Input: part model. Units: mm. Frame: model coordinates. Give positions to 0.01 mm unless a question says otherwise; leave off trailing zeros. Write each loop counter-clockwise with the first axis right and the second up, starting at its lowest first coordinate (ties: lowest second). Pieces come first, ordered by that corner, then holes.
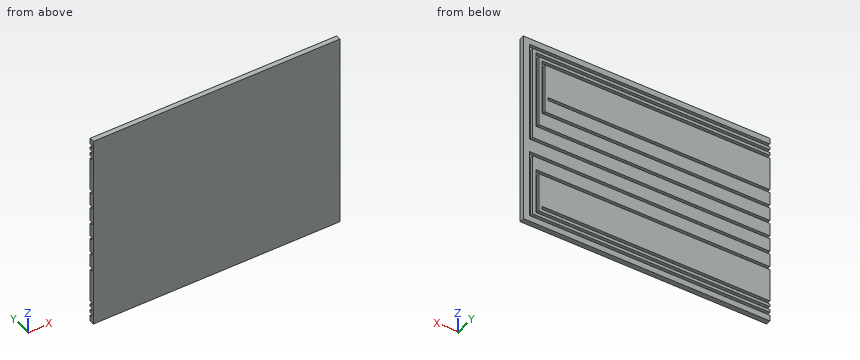
Autodesk Inventor part; units mm, degrees
ref_plane "YZ Plane" through (0, 0, 0) normal (1, 0, 0) x (0, 1, 0)
ref_plane "XZ Plane" through (0, 0, 0) normal (0, 1, 0) x (-1, 0, 0)
ref_plane "XY Plane" through (0, 0, 0) normal (0, 0, 1) x (1, 0, 0)
sketch "Sketch1" plane through (0, 0, 0) normal (0, 1, 0) x (-1, 0, 0)
  line L0 (-135.9557, -16) -> (-525.9557, -16)
  line L1 (-525.9557, -16) -> (-525.9557, 150)
  line L2 (-135.9557, -11) -> (-520.9557, -11)
  line L3 (-520.9557, -11) -> (-520.9557, 145)
  line L4 (-510.9557, 16) -> (-510.9557, 135)
  line L5 (-515.9557, 11) -> (-515.9557, 140)
  line L6 (-500.9557, 43) -> (-500.9557, 125)
  line L7 (-505.9557, 38) -> (-505.9557, 130)
  line L8 (-495.9557, 70) -> (-495.9557, 65)
  line L9 (-535.9557, 160) -> (-135.9557, 160)
  line L10 (-135.9557, 160) -> (-135.9557, -160)
  line L11 (-135.9557, -160) -> (-535.9557, -160)
  line L12 (-535.9557, -160) -> (-535.9557, 160)
  line L13 (-525.9557, -150) -> (-525.9557, -38)
  line L14 (-520.9557, -145) -> (-520.9557, -43)
  line L15 (-510.9557, -135) -> (-510.9557, -70)
  line L16 (-515.9557, -140) -> (-515.9557, -65)
  line L17 (-505.9557, -130) -> (-505.9557, -125)
  line L18 (-525.9557, 150) -> (-135.9557, 150)
  line L19 (-520.9557, 145) -> (-135.9557, 145)
  line L20 (-515.9557, 140) -> (-135.9557, 140)
  line L21 (-505.9557, 130) -> (-135.9557, 130)
  line L22 (-500.9557, 125) -> (-135.9557, 125)
  line L23 (-510.9557, 135) -> (-135.9557, 135)
  line L24 (-135.9557, 70) -> (-495.9557, 70)
  line L25 (-135.9557, 65) -> (-495.9557, 65)
  line L26 (-135.9557, 43) -> (-500.9557, 43)
  line L27 (-135.9557, 38) -> (-505.9557, 38)
  line L28 (-135.9557, 16) -> (-510.9557, 16)
  line L29 (-135.9557, 11) -> (-515.9557, 11)
  line L30 (-525.9557, -38) -> (-135.9557, -38)
  line L31 (-520.9557, -43) -> (-135.9557, -43)
  line L32 (-515.9557, -65) -> (-135.9557, -65)
  line L33 (-510.9557, -70) -> (-135.9557, -70)
  line L34 (-135.9557, -125) -> (-505.9557, -125)
  line L35 (-135.9557, -130) -> (-505.9557, -130)
  line L36 (-135.9557, -135) -> (-510.9557, -135)
  line L37 (-135.9557, -140) -> (-515.9557, -140)
  line L38 (-135.9557, -145) -> (-520.9557, -145)
  line L39 (-135.9557, -150) -> (-525.9557, -150)
  dimension "d2" = 5
  dimension "d6" = 5
  dimension "d13" = 5
  dimension "d17" = 5
  dimension "d23" = 5
  dimension "d24" = 5
  dimension "d30" = 400
  dimension "d31" = 320
  dimension "d35" = 5
  dimension "d40" = 5
  dimension "d43" = 5
  dimension "d46" = 5
  dimension "d52" = 10
  dimension "d53" = 10
extrude "Extrusion1" add sketch "Sketch1" against normal blind 5 contours L10 L30 L13 L39 L11 L12 L9 L18 L1 L0 | L2 L3 L19 L10 L20 L5 L29 | L10 L32 L16 L37 L38 L14 L31 | L28 L4 L23 L10 L21 L7 L27 | L10 L34 L17 L35 L36 L15 L33 | L26 L6 L22 L10 L24 L8 L25
ref_plane "Work Plane2" through (135.9557, 0, 160) normal (0, 0, 1) x (1, 0, 0)
sketch "Sketch3" plane through (135.9557, 0, 160) normal (0, 0, 1) x (1, 0, 0)
  line L0 (0, 0) -> (0, -5)
  line L1 (0, -5) -> (400, -5)
  line L2 (400, -5) -> (400, -8)
  line L3 (400, -8) -> (0, -8)
  line L4 (0, -8) -> (0, -5)
  point P0 (-135.9557, 0)
  dimension "d62" = 3
extrude "Extrusion3" add sketch "Sketch3" against normal blind 320
equation "\"d2\" = d25"
equation "\"d6\" = d26"
equation "\"d13\" = d25"
equation "\"d17\" = d26"
equation "\"d23\" = d25"
equation "\"d24\" = d26"
equation "\"d35\" = d47"
equation "\"d40\" = d47"
equation "\"d43\" = d49"
equation "\"d46\" = d49"
equation "\"d3\" = d25"
equation "\"d4\" = d25"
equation "\"d5\" = d26"
equation "\"d7\" = d25"
equation "\"d8\" = d25"
equation "\"d9\" = d25"
equation "\"d10\" = d26"
equation "\"d12\" = d28"
equation "\"d14\" = d25"
equation "\"d15\" = d28"
equation "\"d16\" = d26"
equation "\"d18\" = d25"
equation "\"d19\" = d25"
equation "\"d20\" = d28"
equation "\"d21\" = d25"
equation "\"d22\" = d25"
equation "\"d25\" = 5"
equation "\"d26\" = 5"
equation "\"d28\" = -1.2 * d25 + 0.2 * d29"
equation "\"d34\" = d47"
equation "\"d36\" = d47"
equation "\"d37\" = d48"
equation "\"d38\" = d47"
equation "\"d39\" = d49"
equation "\"d41\" = d47"
equation "\"d42\" = d48"
equation "\"d44\" = d47"
equation "\"d45\" = d49"
equation "\"d47\" = 5"
equation "\"d48\" = -1.2 * d47 + 0.2 * d50"
equation "\"d49\" = 5"
properties part number "WIRE HOUSING"
Q1. Section B-B, the plane y = -2. Give the number of separate pieces and of enclosed holes in the cut face, then the cut area to 3 significant figures.
Q2. Section A-A, the plane z = -88. Return the cut outline in (x, y).
Q3. Section C-C, the plane z = 118.5. Return the cut outline in (x, y).
Q4. Pin query (flat end, axial travel): pin 1 (2.5 mm diameter, centred on y = -2, z = -128.5, fed in from -X); pin 2 (2.5 mm diameter, centred on x = 336, z = 67, fed in from +Y). Return the tip coordinate at first contact, or that it passes through.
Q5. Material intervals for line 1 along X through (y, z) = (-1, 129); line 2 along X through (y, z) = (-1.25, 22); line 3 along X through (y, z) = (-1.5, 124.5), sorted ascending.
Solutions:
1. separate pieces: 6
1. enclosed holes: 0
1. area: 103,000 mm2
2. outline: (135.96, -8) - (535.96, -8) - (535.96, 0) - (525.96, 0) - (525.96, -5) - (520.96, -5) - (520.96, 0) - (515.96, 0) - (515.96, -5) - (510.96, -5) - (510.96, 0) - (135.96, 0) - close
3. outline: (135.96, -8) - (535.96, -8) - (535.96, 0) - (525.96, 0) - (525.96, -5) - (520.96, -5) - (520.96, 0) - (515.96, 0) - (515.96, -5) - (510.96, -5) - (510.96, 0) - (505.96, 0) - (505.96, -5) - (500.96, -5) - (500.96, 0) - (135.96, 0) - close
4. pin 1: stops at x = 505.96
4. pin 2: stops at y = -5
5. line 1: x = 505.96 to 510.96, 515.96 to 520.96, 525.96 to 535.96
5. line 2: x = 135.96 to 510.96, 515.96 to 520.96, 525.96 to 535.96
5. line 3: x = 135.96 to 500.96, 505.96 to 510.96, 515.96 to 520.96, 525.96 to 535.96
